```python
from build123d import *

# Parameters (mm, degrees)
SKETCH1_R           = 2.54
BOSS_EXTRUDE1_DEPTH = 3.175


with BuildPart() as part:
    # Sketch1 → Boss-Extrude1 (new body)
    with BuildSketch(Plane.XY):
        with BuildLine():
            Line((-101.6, 77.978), (101.6, 77.978))
            ThreePointArc((101.6, 77.978), (105.551312693, 76.341312693), (107.188, 72.39))
            Line((107.188, 72.39), (107.188, 24.765))
            Line((107.188, 24.765), (107.188, -24.765))
            Line((107.188, -24.765), (107.188, -72.39))
            ThreePointArc((107.188, -72.39), (105.551312693, -76.341312693), (101.6, -77.978))
            Line((101.6, -77.978), (-101.6, -77.978))
            ThreePointArc((-101.6, -77.978), (-105.551312693, -76.341312693), (-107.188, -72.39))
            Line((-107.188, -72.39), (-107.188, -24.765))
            Line((-107.188, -24.765), (-107.188, 24.765))
            Line((-107.188, 24.765), (-107.188, 72.39))
            ThreePointArc((-107.188, 72.39), (-105.551312693, 76.341312693), (-101.6, 77.978))
        make_face()
        with Locations((-101.6, 0)):
            Circle(SKETCH1_R, mode=Mode.SUBTRACT)
        with Locations((-50.8, 0)):
            Circle(SKETCH1_R, mode=Mode.SUBTRACT)
        Circle(SKETCH1_R, mode=Mode.SUBTRACT)
        with Locations((101.6, 0)):
            Circle(SKETCH1_R, mode=Mode.SUBTRACT)
        with Locations((50.8, 0)):
            Circle(SKETCH1_R, mode=Mode.SUBTRACT)
        with Locations((-101.6, 72.39)):
            Circle(SKETCH1_R, mode=Mode.SUBTRACT)
        with Locations((0, 72.39)):
            Circle(SKETCH1_R, mode=Mode.SUBTRACT)
        with Locations((101.6, 72.39)):
            Circle(SKETCH1_R, mode=Mode.SUBTRACT)
        with Locations((-101.6, -72.39)):
            Circle(SKETCH1_R, mode=Mode.SUBTRACT)
        with Locations((0, -72.39)):
            Circle(SKETCH1_R, mode=Mode.SUBTRACT)
        with Locations((101.6, -72.39)):
            Circle(SKETCH1_R, mode=Mode.SUBTRACT)
    extrude(amount=BOSS_EXTRUDE1_DEPTH)


solid = part.part
```
Design review of the part built by this model. Coordinates are the model's own, in mm. Coordinates: 2 decimals unless noted, no trailing zeros. Loops run counter-clockwise (first coordinate to the right, second up) from the corner with the lowest first, then second, coordinate; pieces in that order, holes last.
Q1. The part is to be moulded in two halves that separate along Y. For faces 1 (the face through (105.59, -76.3, 1.57)), 2 (the face through (-48.377, 0.763, 1.565)), 3 (the face through (-105.59, 76.3, 1.57)), say which applies: +Y half, -Y half, draft (parallel to the pull), parting line (faces both ways), or undercut.
Reported:
face 1: -Y half
face 2: undercut
face 3: +Y half
Q2. We need section A-A on x = 0. State the section outline as (y, z) points (3 decimals).
Reported:
outline: (-77.978, 0) - (-74.93, 0) - (-74.93, 3.175) - (-77.978, 3.175) - close; (-69.85, 0) - (-2.54, 0) - (-2.54, 3.175) - (-69.85, 3.175) - close; (2.54, 0) - (69.85, 0) - (69.85, 3.175) - (2.54, 3.175) - close; (74.93, 0) - (77.978, 0) - (77.978, 3.175) - (74.93, 3.175) - close
Q3. To check wall thickness, follow line 1 (Y direction, x = 0, z = 1.85); line 2 (Y direction, x = -50.8, z = 0.9). State the ranges of each line that lie inside material, in increasing order.
Reported:
line 1: y = -77.98 to -74.93, -69.85 to -2.54, 2.54 to 69.85, 74.93 to 77.98
line 2: y = -77.98 to -2.54, 2.54 to 77.98
